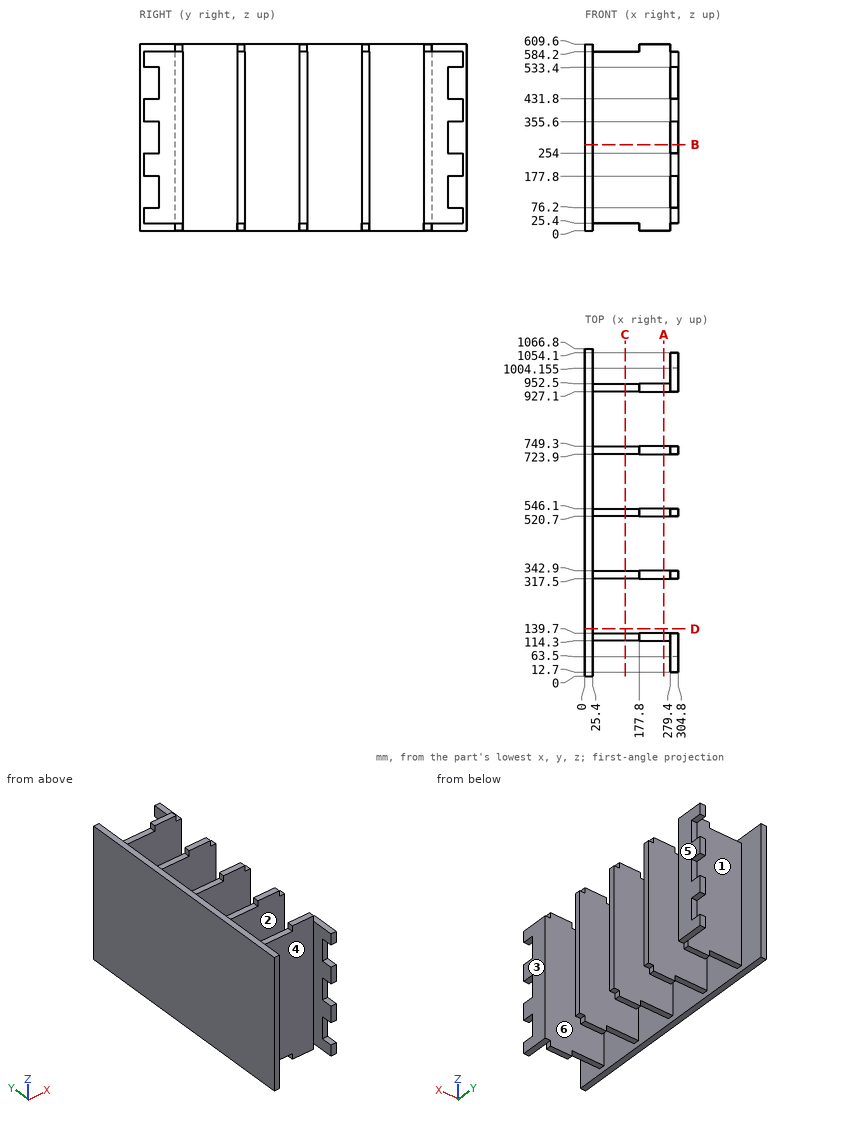
Input: dimensioned drawing with shaded views. Units: mm. Origin: part minimum x, y, z. A direction names the side the tool comes from. Give positions to 0.01 mm unless a question says otherwise; leave off trailing zeros. Loops run counter-clockwise (first coordinate to the right, second up) from the corner with the lowest first, then second, coordinate; pieces in that order, holes last. Notation, with made-up numbers: M 54.25,63.25 L 62.25,63.25 A37 cw 62.25,99.25 Z; hole C -2.75,84.5 d3. An arc over 180 degrees is marked long. Put each result on its own line as item: value. Start each with the question number.
1) Cut plane B-B (z = 281). Output: boundary loops of the cut face in (x, y) (1 decimal).
2) Cut plane A-A (x = 258). Output: boundary loops of the cut face in (y, z).
3) Cut plane D-D (y = 154). Output: boundary loops of the cut face in (x, z).
4) Ray query, line 1 along Y through (x, z) = (42, 424.5); line 2 along X through (y, z) = (212.5, 493.5); line 3 along Z through (x, y) = (154, 139). Return the intervals inside material, ascending.
5) Cut plane C-C (x = 131.5). Output: boundary loops of the cut face in (y, z), then the cut area to 3 significant figures.
6) Pull-direction query (X, two-part tool) for the marked faces 4, 5 and 6; classes: pulls with the +X half, pulls with the -X half, needs draft (parallel to the pull), parting line crosses it, or undercut.
7) Access query for the marked faces 1, 2 and 3. Directions: +Z, -Z, +X, -X, +Y, -Y. A direction counts if a zero-diameter tool reaches every point of the face in a straight line with its end or side. Return the directions, or none.
8) Contact query for flat-ended pins moving along their axis: pin 1 (4 mm diameter, centred on y = 641.5, z = 491, fed in from -X); pin 2 (20.5 mm diameter, centred on x = 294, y = 30, fed in from +Z); pin 3 (20.5 mm diameter, centred on x = 116, y = 944, fed in from -Z); pin 4 (12.5 mm diameter, centred on x = 293, z = 507.5, fed in from -Y). Output: stop coordinate, or through.
Verdict:
1. outline: M 0,0 L 25.4,0 L 25.4,114.3 L 279.4,114.3 L 279.4,63.5 L 304.8,63.5 L 304.8,139.7 L 25.4,139.7 L 25.4,317.5 L 304.8,317.5 L 304.8,342.9 L 25.4,342.9 L 25.4,520.7 L 304.8,520.7 L 304.8,546.1 L 25.4,546.1 L 25.4,723.9 L 304.8,723.9 L 304.8,749.3 L 25.4,749.3 L 25.4,927.1 L 304.8,927.1 L 304.8,1004.2 L 279.4,1004.2 L 279.4,952.5 L 25.4,952.5 L 25.4,1066.8 L 0,1066.8 Z
2. outline: M 114.3,0 L 139.7,0 L 139.7,609.6 L 114.3,609.6 Z; M 317.5,0 L 342.9,0 L 342.9,609.6 L 317.5,609.6 Z; M 520.7,0 L 546.1,0 L 546.1,609.6 L 520.7,609.6 Z; M 723.9,0 L 749.3,0 L 749.3,609.6 L 723.9,609.6 Z; M 927.1,0 L 952.5,0 L 952.5,609.6 L 927.1,609.6 Z
3. outline: M 0,0 L 25.4,0 L 25.4,609.6 L 0,609.6 Z
4. line 1: 114.3 to 139.7, 317.5 to 342.9, 520.7 to 546.1, 723.9 to 749.3, 927.1 to 952.5
4. line 2: 0 to 25.4
4. line 3: 25.4 to 584.2
5. outline: M 114.3,25.4 L 139.7,25.4 L 139.7,584.2 L 114.3,584.2 Z; M 317.5,25.4 L 342.9,25.4 L 342.9,584.2 L 317.5,584.2 Z; M 520.7,25.4 L 546.1,25.4 L 546.1,584.2 L 520.7,584.2 Z; M 723.9,25.4 L 749.3,25.4 L 749.3,584.2 L 723.9,584.2 Z; M 927.1,25.4 L 952.5,25.4 L 952.5,584.2 L 927.1,584.2 Z
5. area: 71,000 mm2
6. face 4: undercut
6. face 5: pulls with the +X half
6. face 6: needs draft
7. face 1: +Z, -Z, +Y
7. face 2: +Z, -Z, +X
7. face 3: +Z, -Z, +X, +Y, -Y
8. pin 1: x = 0
8. pin 2: z = 584.2
8. pin 3: z = 25.4
8. pin 4: y = 63.5
